Check sheet for the modelled part. Datum: model origin and axes. Units: mm. A direction names the side the tool comes from. Coordinates: 2 decimals unless noted, no trailing zeros. Write each loop counter-clockwise with the first axis right and the second up, starting at its lowest first coordinate (ties: lowest second). Pieces come first, ordered by that corner, then holes. Notation, with made-up numbers: (16.5, 2) -> (40.5, 2) arc R26 ccw to (40.5, 33) -> close; hole circle Ø5 at (-4.75, 63.25). An arc over 180 degrees is marked (long way). One line per item, written item: value. Start each with the question number.
1) Sectioned sample at A-A on z = 1.8. Enter the section's corners in (x, y) (3 decimals).
2) Set-up check for faces 1 (the flat face through (8.4, 2.4, -8.4)), 2 (the cylindrical face through (-0.143, -0.937, 2.253)): record each of +Z, -Z, +X, -X, +Y, -Y from which the full face is reachable in a straight line by a thin tool's end or side.
3) Sectioned sample at D-D on x = -6.5. Enter the section's corners in (y, z), plus the area to 3 significant figures.
4) Scan line: line 1 along Y through (x, z) = (4, 0.5). Record every from-to range of solid material in increasing order. Write a range as [from, to].
5) Sectioned sample at B-B on x = 0. Enter the section's corners in (y, z) (3 decimals), plus the area to 3 significant figures.
6) Sectioned sample at C-C on y = -0.75. Enter the section's corners in (x, z) (3 decimals), plus the area to 3 significant figures.
7) Gauge pin test, flat ends, axial feed: P1, Ø4, axis at x = -4, z = 3, coming from the -Y side; P2, Ø10, axis at x = 1, z = 0, coming from the -Y side. Record the tip position at first contact, or that the pin passes through.
```python
from build123d import *

# Parameters (mm, degrees)
BOSS_EXTRUDE1_DEPTH = 4.8
FILLET1_R           = 0.5
SKETCH2_R           = 0.475
BOSS_EXTRUDE2_DEPTH = 1.9


with BuildPart() as part:
    # Sketch1 → Boss-Extrude1 (new body)
    with BuildSketch(Plane(origin=(0, 0, 0), x_dir=(1, 0, 0), z_dir=(0, 1, 0))):
        Polygon((9.15, 7.65), (7.65, 9.15), (-9.15, 9.15), (-9.15, -9.15), (9.15, -9.15), align=None)
    extrude(amount=BOSS_EXTRUDE1_DEPTH)

    # Fillet1
    fillet1_edges = [part.edges().sort_by_distance(p)[0] for p in [
        (-9.15, 2.4, 9.15),
        (-9.15, 2.4, -9.15),
        (9.15, 2.4, 9.15),
    ]]
    fillet(fillet1_edges, radius=FILLET1_R)

    # Sketch2 → Boss-Extrude2 (add)
    with BuildSketch(Plane.XZ):
        with Locations(Location((0, 1.8, 0), (0, 0, 90))):  # turned: the seam where the file's is
            Circle(SKETCH2_R)
    extrude(amount=BOSS_EXTRUDE2_DEPTH)


solid = part.part
```
Answers:
1. outline: (-9.15, 0) -> (-0.475, 0) -> (-0.475, -1.9) -> (0.475, -1.9) -> (0.475, 0) -> (9.15, 0) -> (9.15, 4.8) -> (-9.15, 4.8) -> close
2. face 1: -Z, +X, +Y, -Y
2. face 2: -Y
3. outline: (0, -9.15) -> (4.8, -9.15) -> (4.8, 9.15) -> (0, 9.15) -> close
3. area: 87.8 mm2
4. line 1: y = [0, 4.8]
5. outline: (-1.9, 1.325) -> (0, 1.325) -> (0, -9.15) -> (4.8, -9.15) -> (4.8, 9.15) -> (0, 9.15) -> (0, 2.275) -> (-1.9, 2.275) -> close
5. area: 89.6 mm2
6. outline: circle Ø0.95 at (0, 1.8)
6. area: 0.709 mm2
7. P1: stops at y = 0
7. P2: stops at y = -1.9
